Design review of the part built by this model. Coordinates are the model's own, in mm. A direction names the side the tool comes from. Give positions to 0.01 mm unless a question says otherwise; leave off trailing zeros. Loops run counter-clockwise (first coordinate to the right, second up) from the corner with the lowest first, then second, coordinate; pieces in that order, holes last. Notation, with made-up numbers: M 10.25,43 L 47.25,43 A16 ccw 47.25,72 Z; hole C -9,-25 d3. An arc over 180 degrees is marked long. Use a Markdown table: item, result. Add a question column.
(1) Add section C-C, the plane x = -195. Give the boundary of the cut face in (y, z).
(2) For probe 1 along X at (y, z) = (0, -12.5); probe 2 along X at (y, z) = (2.5, -14); probe 3 along Z at (x, y) = (61, 2), list the stretches that pass through material, from the lowest coordinate up.
(3) For faces 4 (the face through (-195, 0, 0)), 5 (the face through (-350, 0, 0)), list the 3-axis set-ups (+Z, -Z, +X, -X, +Y, -Y) from which the entire face can be reached by the end or side of a thin tool; tool diameter is ignored.
(4) Add section A-A, the plane x = 97. Give the boundary of the cut face in (y, z), then the cut area to 3 significant figures.
(5) Draft analysis for pull direction Y (two halves, no side actions). For faces 1 (the face through (195, 0, 0)), 2 (the face through (350, 0, 0)), 3 (the face through (4.9, 9.229, -17.743)), state which applies: pulls with the +Y half, pulls with the -Y half, needs draft (parallel to the pull), parting line crosses it, or undercut.
(6) Insertion check: pin 1 Ø17.5 at (x, y) = (195, 0) entering from +Z; pin 2 Ø6 at (x, y) = (-261, -5) entering from -Z; pin 3 Ø12 at (x, y) = (-197, -11) entering from +Z. Each pin has a flat end and moves straight along its axis. Give the tip position at first contact, or say it passes through.
(7) Add section B-B, the plane z = -7. State how many separate pieces and enclosed holes the cut face has, then the cut area to 3 significant figures.
```python
from build123d import *

# Parameters (mm, degrees)
F1_DEPTH = 350
F2_R     = 11
F3_DEPTH = 25.4
F5_R     = 3
F6_DEPTH = 47.3215082123


with BuildPart() as f1:
    # F0 (on Right) → F1 (new body, symmetric)
    with BuildSketch(Plane.YZ):
        with BuildLine():
            ThreePointArc((10, 17.3205080757), (-17.3205080757, -10), (20, 0))
            ThreePointArc((20, 0), (17.3205080757, 10), (10, 17.3205080757))
        make_face()
    extrude(amount=F1_DEPTH, both=True)

    # F2 (on Top) → F3 (cut)
    with BuildSketch(Plane.XY):
        with Locations((-195, 0)):
            Circle(F2_R)
        with Locations((195, 0)):
            Circle(F2_R)
    extrude(amount=-F3_DEPTH, mode=Mode.SUBTRACT)

    # F5 (on face) → F6 (cut, through all)
    with BuildSketch(Plane(origin=(0, 10, 17.3205080757), x_dir=(1, 0, 0), z_dir=(0, 0.5, 0.8660254038))):
        Circle(F5_R)
    extrude(amount=-F6_DEPTH, mode=Mode.SUBTRACT)


solid = f1.part
```
Established:
| question | item | result |
|---|---|---|
| 1 | outline | M -11,-16.7 L -11,0 L 11,0 L 11,-16.7 A20 ccw long Z |
| 2 | probe 1 | -350 to -206, -184 to 184, 206 to 350 |
| 2 | probe 2 | -350 to -205.71, -184.29 to 184.29, 205.71 to 350 |
| 2 | probe 3 | -19.9 to 19.9 |
| 3 | face 4 | -Z |
| 3 | face 5 | +Z, -Z, -X, +Y, -Y |
| 4 | outline | C 0,0 d40 |
| 4 | area | 1,260 mm^2 |
| 5 | face 1 | undercut |
| 5 | face 2 | needs draft |
| 5 | face 3 | parting line crosses it |
| 6 | pin 1 | z = 20 |
| 6 | pin 2 | z = -19.9 |
| 6 | pin 3 | z = 19.36 |
| 7 | separate pieces | 1 |
| 7 | enclosed holes | 3 |
| 7 | area | 25,400 mm^2 |
